Part model, mm, in its own coordinate system. A direction names the side the tool comes from. Coordinates: 2 decimals unless noted, no trailing zeros. Loops run counter-clockwise (first coordinate to the right, second up) from the corner with the lowest first, then second, coordinate; pieces in that order, holes last. Notation, with made-up numbers: M 54.5,-3 L 86.5,-3 A21 cw 86.5,29 Z; hole C 57.5,66.5 d7. An arc over 180 degrees is marked long. Use a Markdown table: item, result. Add a question column.
1) Band-saw the part on C-C (z = 24.5). List the corners of the cut face in (x, y).
2) Tool access for faces 4 (the cylindrical face through (-13.605, -5.044, -9.41)), 5 (the flat face through (0, -7.62, 4)): list every direction of +Z, -Z, +X, -X, +Y, -Y with a clear straight run to the whole face (end or side of a thin tool).
3) Band-saw the part on D-D (z = 14.5). List the corners of the cut face in (x, y), plus the area to 3 significant figures.
4) Band-saw the part on A-A (y = -6). List the corners of the cut face in (x, z) (3 decimals), plus the area to 3 significant figures.
5) Band-saw the part on B-B (x = 0). List the corners of the cut face in (y, z).
6) Wall check: probe 1 along Z at (x, y) = (-8, -2.75); probe 2 along Z at (x, y) = (-8.5, -6); probe 3 along Y at (x, z) = (23, 3.5). Give the ranges that are in metal, low to high. Write a range as from..to.
7) Pull direction X, two halves, no side cores. Call faces 1 (the flat face through (-14.3, -7.62, 25.2)), 2 (the cylindrical face through (-25.394, -5.044, 3.383)), 3 (the cylindrical face through (-6.88, -3.76, -27.07)): released by +X, released by -X, zero draft, split by the parting line, or undercut.
8) Pin check, flat tips, straight feed: pin 1 Ø12 at (x, z) = (-17.5, 11.5) entering from +Y; pin 2 Ø1.5 at (x, y) = (15, -5) entering from +Z; pin 3 Ø1.5 at (x, y) = (-16.5, -6) entering from -Z; pin 4 Ø3 at (y, z) = (-6, -19.5) entering from -X. Stop position of each tip, or through.
from build123d import *

# Parameters (mm, degrees)
F0_R     = 31.75
F1_DEPTH = 7.62
F2_DEPTH = 2.54


with BuildPart() as f1:
    # F0 (on Front) → F1 (new body)
    with BuildSketch(Plane.XZ):
        with Locations((0, 3.923906)):
            Circle(F0_R)
        with BuildLine():
            ThreePointArc((-1.27, 29.292136), (0, 29.323906), (1.27, 29.292136))
            ThreePointArc((1.27, 29.292136), (25.4, 3.923906), (1.27, -21.444324))
            ThreePointArc((1.27, -21.444324), (0, -21.476094), (-1.27, -21.444324))
            ThreePointArc((-1.27, -21.444324), (-25.4, 3.923906), (-1.27, 29.292136))
        make_face(mode=Mode.SUBTRACT)
        with BuildLine():
            ThreePointArc((1.27, -1.648196), (5.715, 3.923906), (1.27, 9.496008))
            ThreePointArc((1.27, 9.496008), (0, 9.638906), (-1.27, 9.496008))
            ThreePointArc((-1.27, 9.496008), (-5.715, 3.923906), (-1.27, -1.648196))
            ThreePointArc((-1.27, -1.648196), (0, -1.791094), (1.27, -1.648196))
        make_face()
        with BuildLine():
            ThreePointArc((19.00762, 5.193906), (13.470384, 17.39429), (1.27, 22.931525))
            ThreePointArc((1.27, 22.931525), (0, 22.973906), (-1.27, 22.931525))
            ThreePointArc((-1.27, 22.931525), (-13.470384, 17.39429), (-19.00762, 5.193906))
            Line((-19.00762, 5.193906), (-9.439954, 5.193906))
            ThreePointArc((-9.439954, 5.193906), (-6.735192, 10.659098), (-1.27, 13.36386))
            ThreePointArc((-1.27, 13.36386), (0, 13.448906), (1.27, 13.36386))
            ThreePointArc((1.27, 13.36386), (6.735192, 10.659098), (9.439954, 5.193906))
            Line((9.439954, 5.193906), (19.00762, 5.193906))
        make_face()
        with BuildLine():
            ThreePointArc((1.27, -15.083714), (13.470384, -9.546478), (19.00762, 2.653906))
            Line((19.00762, 2.653906), (9.439954, 2.653906))
            ThreePointArc((9.439954, 2.653906), (6.735192, -2.811286), (1.27, -5.516048))
            ThreePointArc((1.27, -5.516048), (0, -5.601094), (-1.27, -5.516048))
            ThreePointArc((-1.27, -5.516048), (-6.735192, -2.811286), (-9.439954, 2.653906))
            Line((-9.439954, 2.653906), (-19.00762, 2.653906))
            ThreePointArc((-19.00762, 2.653906), (-13.470384, -9.546478), (-1.27, -15.083714))
            ThreePointArc((-1.27, -15.083714), (0, -15.126094), (1.27, -15.083714))
        make_face()
    extrude(amount=F1_DEPTH)

    # F0 (on Front) → F2 (join)
    with BuildSketch(Plane.XZ):
        with BuildLine():
            ThreePointArc((-19.00762, 5.193906), (-13.470384, 17.39429), (-1.27, 22.931525))
            Line((-1.27, 22.931525), (-1.27, 29.292136))
            ThreePointArc((-1.27, 29.292136), (-25.4, 3.923906), (-1.27, -21.444324))
            Line((-1.27, -21.444324), (-1.27, -15.083714))
            ThreePointArc((-1.27, -15.083714), (-13.470384, -9.546478), (-19.00762, 2.653906))
            ThreePointArc((-19.00762, 2.653906), (-19.05, 3.923906), (-19.00762, 5.193906))
        make_face()
        with BuildLine():
            Line((1.27, 29.292136), (1.27, 22.931525))
            ThreePointArc((1.27, 22.931525), (13.470384, 17.39429), (19.00762, 5.193906))
            ThreePointArc((19.00762, 5.193906), (19.05, 3.923906), (19.00762, 2.653906))
            ThreePointArc((19.00762, 2.653906), (13.470384, -9.546478), (1.27, -15.083714))
            Line((1.27, -15.083714), (1.27, -21.444324))
            ThreePointArc((1.27, -21.444324), (25.4, 3.923906), (1.27, 29.292136))
        make_face()
        with BuildLine():
            ThreePointArc((19.00762, 2.653906), (19.05, 3.923906), (19.00762, 5.193906))
            Line((19.00762, 5.193906), (9.439954, 5.193906))
            ThreePointArc((9.439954, 5.193906), (6.735192, 10.659098), (1.27, 13.36386))
            Line((1.27, 13.36386), (1.27, 9.496008))
            ThreePointArc((1.27, 9.496008), (5.715, 3.923906), (1.27, -1.648196))
            Line((1.27, -1.648196), (1.27, -5.516048))
            ThreePointArc((1.27, -5.516048), (6.735192, -2.811286), (9.439954, 2.653906))
            Line((9.439954, 2.653906), (19.00762, 2.653906))
        make_face()
        with BuildLine():
            Line((-9.439954, 5.193906), (-19.00762, 5.193906))
            ThreePointArc((-19.00762, 5.193906), (-19.05, 3.923906), (-19.00762, 2.653906))
            Line((-19.00762, 2.653906), (-9.439954, 2.653906))
            ThreePointArc((-9.439954, 2.653906), (-6.735192, -2.811286), (-1.27, -5.516048))
            Line((-1.27, -5.516048), (-1.27, -1.648196))
            ThreePointArc((-1.27, -1.648196), (-5.715, 3.923906), (-1.27, 9.496008))
            Line((-1.27, 9.496008), (-1.27, 13.36386))
            ThreePointArc((-1.27, 13.36386), (-6.735192, 10.659098), (-9.439954, 5.193906))
        make_face()
        with BuildLine():
            ThreePointArc((-1.27, 22.931525), (0, 22.973906), (1.27, 22.931525))
            Line((1.27, 22.931525), (1.27, 29.292136))
            ThreePointArc((1.27, 29.292136), (0, 29.323906), (-1.27, 29.292136))
            Line((-1.27, 29.292136), (-1.27, 22.931525))
        make_face()
        with BuildLine():
            Line((1.27, 9.496008), (1.27, 13.36386))
            ThreePointArc((1.27, 13.36386), (0, 13.448906), (-1.27, 13.36386))
            Line((-1.27, 13.36386), (-1.27, 9.496008))
            ThreePointArc((-1.27, 9.496008), (0, 9.638906), (1.27, 9.496008))
        make_face()
        with BuildLine():
            ThreePointArc((-1.27, -5.516048), (0, -5.601094), (1.27, -5.516048))
            Line((1.27, -5.516048), (1.27, -1.648196))
            ThreePointArc((1.27, -1.648196), (0, -1.791094), (-1.27, -1.648196))
            Line((-1.27, -1.648196), (-1.27, -5.516048))
        make_face()
        with BuildLine():
            ThreePointArc((-1.27, -21.444324), (0, -21.476094), (1.27, -21.444324))
            Line((1.27, -21.444324), (1.27, -15.083714))
            ThreePointArc((1.27, -15.083714), (0, -15.126094), (-1.27, -15.083714))
            Line((-1.27, -15.083714), (-1.27, -21.444324))
        make_face()
    extrude(amount=F2_DEPTH)


solid = f1.part
Entries:
| question | item | result |
|---|---|---|
| 1 | outline | M -24.18,-7.62 L -14.89,-7.62 L -14.89,-2.54 L 14.89,-2.54 L 14.89,-7.62 L 24.18,-7.62 L 24.18,0 L -24.18,0 Z |
| 2 | face 4 | -Y |
| 2 | face 5 | +Z, -Z, +X, -X, -Y |
| 3 | outline | M -29.94,-7.62 L -23.09,-7.62 L -23.09,-2.54 L -15.84,-2.54 L -15.84,-7.62 L 15.84,-7.62 L 15.84,-2.54 L 23.09,-2.54 L 23.09,-7.62 L 29.94,-7.62 L 29.94,0 L -29.94,0 Z |
| 3 | area | 383 mm2 |
| 4 | outline | C 0,3.924 d63.5; M -19.008,2.654 A19.05 ccw -1.27,-15.084 A19.05 ccw 1.27,-15.084 A19.05 ccw 19.008,2.654 L 9.44,2.654 A9.525 cw 1.27,-5.516 A9.525 cw -1.27,-5.516 A9.525 cw -9.44,2.654 Z; M -19.008,5.194 L -9.44,5.194 A9.525 cw -1.27,13.364 A9.525 cw 1.27,13.364 A9.525 cw 9.44,5.194 L 19.008,5.194 A19.05 ccw 1.27,22.932 A19.05 ccw -1.27,22.932 A19.05 ccw Z; M -1.27,-1.648 A5.715 ccw 1.27,-1.648 A5.715 ccw 1.27,9.496 A5.715 ccw -1.27,9.496 A5.715 ccw Z; hole M -1.27,-21.444 A25.4 ccw 1.27,-21.444 A25.4 ccw 1.27,29.292 A25.4 ccw -1.27,29.292 A25.4 ccw Z |
| 4 | area | 2,050 mm2 |
| 5 | outline | M -7.62,-27.83 L 0,-27.83 L 0,35.67 L -7.62,35.67 L -7.62,29.32 L -2.54,29.32 L -2.54,22.97 L -7.62,22.97 L -7.62,13.45 L -2.54,13.45 L -2.54,9.64 L -7.62,9.64 L -7.62,-1.79 L -2.54,-1.79 L -2.54,-5.6 L -7.62,-5.6 L -7.62,-15.13 L -2.54,-15.13 L -2.54,-21.48 L -7.62,-21.48 Z |
| 6 | probe 1 | -26.8..-20.18, -13.36..-1.25, 9.09..21.21, 28.03..34.65 |
| 6 | probe 2 | -26.67..-20.01, -13.12..-0.37, 8.22..20.97, 27.86..34.51 |
| 6 | probe 3 | -2.54..0 |
| 7 | face 1 | zero draft |
| 7 | face 2 | undercut |
| 7 | face 3 | split by the parting line |
| 8 | pin 1 | y = 0 |
| 8 | pin 2 | z = 32.3 |
| 8 | pin 3 | z = -23.64 |
| 8 | pin 4 | x = -22.97 |
